```python
from build123d import *


with BuildPart() as f1:
    # F0 (on Front) → F1 (revolve)
    with BuildSketch(Plane.XZ):
        with BuildLine():
            Line((0, 50.8), (0, 0))
            Line((0, 0), (31.75, 0))
            Line((31.75, 0), (31.75, 4.7625))
            ThreePointArc((31.75, 4.7625), (20.214433, 14.109899), (15.875, 28.30893))
            Line((15.875, 28.30893), (15.875, 50.8))
            Line((15.875, 50.8), (0, 50.8))
        make_face()
    revolve(axis=Axis((0, 0, 25.4), (0, 0, -1)))

    # F2 (on face) → F5 section 0
    with BuildSketch(Plane.XY.offset(50.8)):
        Polygon((3.28782, 7.9375), (-3.28782, 7.9375), (-7.9375, 3.28782), (-7.9375, -3.28782), (-3.28782, -7.9375), (3.28782, -7.9375), (7.9375, -3.28782), (7.9375, 3.28782), align=None)
    # F4 (on offset) → F5 section 1
    with BuildSketch(Plane.XY.offset(34.925)):
        Polygon((2.630256, 6.35), (-2.630256, 6.35), (-6.35, 2.630256), (-6.35, -2.630256), (-2.630256, -6.35), (2.630256, -6.35), (6.35, -2.630256), (6.35, 2.630256), align=None)
    loft(mode=Mode.SUBTRACT)


solid = f1.part
```
Can you work these out from the model? Positions are in its coordinate system, mm. A direction names the side the tool comes from. Coordinates: 2 decimals unless noted, no trailing zeros. Write each loop counter-clockwise with the first axis right and the second up, starting at its lowest first coordinate (ties: lowest second). Pieces come first, ordered by that corner, then holes. Notation, with made-up numbers: (-37.5, 49.25) - (0.5, 49.25) arc R32 cw to (0.5, 83.25) - close; hole circle Ø8 at (1, 24.25). An arc over 180 degrees is marked (long way). Return JSON: item names as keys, results as strings.
Q1. If we section it at A-A (z = 31.5): Please give me the cut outline in (x, y) (3 decimals).
Computed values:
{"outline": "circle Ø31.75 at (0, 0)"}
Q2. On a 3-axis mill with a long thin cutter (end or side, diameter ignored), from which of +Z, -Z, +X, -X, +Y, -Y can I reach the whole of each face in a straight line? I mean faces 4 (the flat face through (7, 7, 50.8)), 5 (the cylindrical face through (-3.441, 15.497, 39.712)). Say none if no direction works.
Computed values:
{"face 4": "+Z, +X, -X, +Y, -Y", "face 5": "+Z"}
Q3. If we section it at B-B (z = 11.5): Please give me the cut outline in (x, y), then the cut area to 3 significant figures.
Computed values:
{"outline": "circle Ø44.46 at (0, 0)", "area": "1,550 mm2"}
Q4. Thinking about a two-plate mould opening in X: for faces 1 (the flat face through (0, 0, 34.925)), 2 (the flat face through (0, 0, 0)), 3 (the cylindrical face through (-6.883, 30.995, 2.415)), which applies, +X half, -X half, draft (parallel to the pull), parting line (faces both ways), or undercut?
Computed values:
{"face 1": "undercut", "face 2": "draft", "face 3": "parting line"}
Q5. Please list where these lines run through material, in increasing order: L1, parallel to Y at x = -0.5, z = 33.5; L2, parallel to Y at x = -18, z = 7.5; L3, parallel to X at y = 5, z = 32.5. Write a range as from..to.
Computed values:
{"L1": "y = -15.87..15.87", "L2": "y = -19.73..19.73", "L3": "x = -15.07..15.07"}
Q6. I'm going to push flat-ended pins straight in: pin 1 Ø5 at (y, z) = (2.5, 13) entering from +X; pin 2 Ø3 at (y, z) = (11.5, 39) entering from +X; pin 3 Ø8 at (y, z) = (5, 11.5) entering from -X. Where does each tip first touch, or does it pass through?
Computed values:
{"pin 1": "stops at x = 23.04", "pin 2": "stops at x = 12.33", "pin 3": "stops at x = -26.28"}
